Build history of the part. All positions in model axes, mm. Face numbers are marked on the shaded views. A direction names the side the tool comes from. Coordinates: 2 decimals unless noted, no trailing zeros. Write each loop counter-clockwise with the first axis right and the second up, starting at its lowest first coordinate (ties: lowest second). Pieces come first, ordered by that corner, then holes.
```python
from build123d import *

# Parameters (mm, degrees)
SKETCH_2_R          = 1.6
CUT_EXTRUDE_1_DEPTH = 10
SKETCH_3_R          = 1.6
CUT_EXTRUDE_2_DEPTH = 10
FILLET_1_R          = 2


with BuildPart() as part:
    # 草图1 → 旋转1 (revolve)
    with BuildSketch(Plane.XY, mode=Mode.PRIVATE) as revolve_1_sk:
        with BuildLine():
            Line((4.67441793, 1.645613509), (5.265095642, 0))
            Line((5.265095642, 0), (21.265095642, 0))
            Line((21.265095642, 0), (21.265095642, 2.244719328))
            Line((21.265095642, 2.244719328), (14.3, 2.244719328))
            Line((14.3, 2.244719328), (8.034357928, 2.244719328))
            Line((8.034357928, 2.244719328), (6.321891904, 2.244719328))
            Line((6.321891904, 2.244719328), (5.629770002, 4.172953844))
            Line((5.629770002, 4.172953844), (6.556827402, 4.172953844))
            Line((6.556827402, 4.172953844), (5.659767787, 12.454719003))
            Line((5.659767787, 12.454719003), (6.321891904, 12.454719003))
            Line((6.321891904, 12.454719003), (5.315776989, 21.743296168))
            Line((5.315776989, 21.743296168), (5.894592711, 21.743296168))
            Line((5.894592711, 21.743296168), (4.963884004, 29.092954865))
            Line((4.963884004, 29.092954865), (5.315776989, 29.092954865))
            Line((5.315776989, 29.092954865), (4.963884004, 31.909590534))
            Line((4.963884004, 31.909590534), (4.001695177, 31.909590534))
            Line((4.001695177, 31.909590534), (4.557178871, 2.283793527))
            ThreePointArc((4.557178871, 2.283793527), (4.589745294, 1.959917343), (4.67441793, 1.645613509))
        make_face()
    revolve(revolve_1_sk.sketch.rotate(Axis((0, 0, 0), (0, 1, 0)), 90), axis=Axis((0, 0, 0), (0, 1, 0)))

    # 草图2 → 切除-拉伸1 (cut)
    with BuildSketch(Plane.XZ):
        with Locations(Location((-16, 0, 0), (0, 0, 270))):
            Circle(SKETCH_2_R)
        with Locations(Location((0, -16, 0), (0, 0, 270))):
            Circle(SKETCH_2_R)
        with Locations(Location((16, 0, 0), (0, 0, 270))):
            Circle(SKETCH_2_R)
        with Locations(Location((0, 16, 0), (0, 0, 270))):
            Circle(SKETCH_2_R)
    extrude(amount=-CUT_EXTRUDE_1_DEPTH, mode=Mode.SUBTRACT)

    # 草图3 → 切除-拉伸2 (cut)
    with BuildSketch(Plane(origin=(0, 2.244719328, 0), x_dir=(1, 0, 0), z_dir=(0, 1, 0))):
        with BuildLine():
            ThreePointArc((-7.531954162, 19.886527076), (-21.265095642, 0), (-7.531954162, -19.886527076))
            Line((-7.531954162, -19.886527076), (-7.531954162, 19.886527076))
        make_face()
        with Locations((-16, 0)):
            Circle(SKETCH_3_R, mode=Mode.SUBTRACT)
    extrude(amount=-CUT_EXTRUDE_2_DEPTH, mode=Mode.SUBTRACT)

    # 圆角1
    fillet_1_edges = [part.edges().sort_by_distance(p)[0] for p in [
        (-7.531954162, 1.122359664, 19.886527076),
        (-7.531954162, 1.122359664, -19.886527076),
    ]]
    fillet(fillet_1_edges, radius=FILLET_1_R)


solid = part.part
```
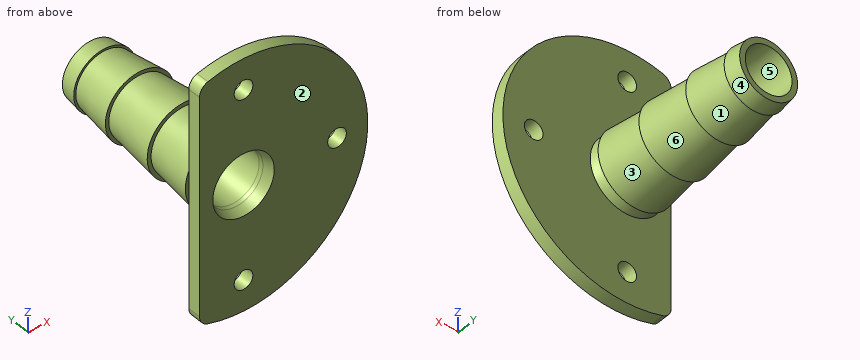
1. Saw through at A-A on x = 16. List the corners of the cut face in (y, z), plus the area to 3 significant figures.
Computed values:
outline: (0, -14.01) - (2.24, -14.01) - (2.24, -1.6) - (0, -1.6) - close; (0, 1.6) - (2.24, 1.6) - (2.24, 14.01) - (0, 14.01) - close
area: 55.7 mm2
2. Saw through at B-B on z = 15. List the corners of the cut face in (x, y), plus the area to 3 significant figures.
Computed values:
outline: (-7.53, 0) - (-1.25, 0) - (-1.25, 2.24) - (-7.53, 2.24) - close; (1.25, 0) - (15.07, 0) - (15.07, 2.24) - (1.25, 2.24) - close
area: 45.1 mm2
3. Flat gauge pins, fed straight in: pin 1 (3 mm diameter, centred on y = 6.5, z = 0, fed in from +X); pin 2 (8.5 mm diameter, centred on x = 12.5, z = -4, fed in from +Y); pin 3 (8 mm diameter, centred on y = 23.5, z = 2.5, fed in from +X). Where does each tip first touch, or does it go through?
Computed values:
pin 1: stops at x = 6.47
pin 2: stops at y = 2.24
pin 3: stops at x = 5.89
4. Saw through at C-C on y = 10. List the corners of the cut face in (x, z) (1 decimal), plus the area to 3 significant figures.
Computed values:
outline: circle Ø11.9 at (0, 0); hole circle Ø8.8 at (0, 0)
area: 49.1 mm2
5. Mould opens along Y. For the marked faces 3, 4, 5 and 6 say: +Y half, -Y half, draft (parallel to the pull), parting line (faces both ways), or undercut.
Computed values:
face 3: undercut
face 4: +Y half
face 5: -Y half
face 6: undercut
6. 3-axis set-ups, long thin cutter, end or side, ignore diameter. For the marked faces 1 and 2: which of +Z, -Z, +X, -X, +Y, -Y reach the whole face in a straight line?
Computed values:
face 1: none
face 2: +Z, -Z, +X, -X, -Y
7. Probe line 1 along X through (y, z) = (1.15, 0); line 2 along X through (y, z) = (1.4, 0); line 3 along Y through (x, z) = (13.25, -14.5). List the from-to ranges inside material, lowest first.
Computed values:
line 1: x = -7.53 to -4.85, 4.85 to 14.4, 17.6 to 21.27
line 2: x = -7.53 to -4.76, 4.76 to 14.4, 17.6 to 21.27
line 3: y = 0 to 2.24
8. Saw through at D-D on z = 0. State how many separate pieces and enclosed holes the cut face has, plus the area to 3 significant figures.
Computed values:
separate pieces: 3
enclosed holes: 0
area: 123 mm2
